Autodesk Inventor part; units mm, degrees
ref_plane "YZ Plane" through (0, 0, 0) normal (1, 0, 0) x (0, 1, 0)
ref_plane "XZ Plane" through (0, 0, 0) normal (0, 1, 0) x (-1, 0, 0)
ref_plane "XY Plane" through (0, 0, 0) normal (0, 0, 1) x (1, 0, 0)
sketch "Sketch1" plane through (0, 0, 0) normal (0, 0, 1) x (1, 0, 0)
  circle A0 centre (0, 0) radius 36
  dimension "d0" = 72
extrude "Extrusion1" add sketch "Sketch1" along normal blind 2
sketch "Sketch2" plane through (0, 0, 2) normal (0, 0, 1) x (1, 0, 0)
  circle A0 centre (0, 0) radius 36
  circle A1 centre (0, 0) radius 34
  dimension "d3" = 2
extrude "Extrusion2" add sketch "Sketch2" along normal blind 4
sketch "Sketch4" plane through (0, 0, 2) normal (0, 0, 1) x (1, 0, 0)
  point P0 (0, 0)
  point P1 (0, 0)
hole "Hole1" at (0, 0, 2) direction (0, 0, -1) diameter 10.1 end through all
sketch "Sketch5" plane through (0, 0, 2) normal (0, 0, 1) x (1, 0, 0)
  point P0 (0, 0)
  point P1 (0, 22.5)
  dimension "d13" = 22.5
hole "Hole2" at (0, 22.5, 2) direction (0, 0, -1) diameter 5.3 end through all
pattern_circular "Circular Pattern1" count 5 over 360 about axis through (0, 0, -100) along (0, 0, 1) of "Hole2"
sketch "Sketch8" plane through (0, 0, 2) normal (0, 0, 1) x (1, 0, 0)
  circle A0 centre (21.3988, 6.9529) radius 2.65
  circle A1 centre (13.2252, -18.2029) radius 2.65
  circle A2 centre (-13.2252, -18.2029) radius 2.65
  circle A3 centre (-21.3988, 6.9529) radius 2.65
  circle A4 centre (0, 22.5) radius 2.65
  circle A5 centre (0, 0) radius 5.05
  circle A6 centre (0, 0) radius 34
  line L0 (-2, 15) -> (2, 15)
  line L1 (2, 15) -> (2, 7)
  line L2 (2, 7) -> (-2, 7)
  line L3 (-2, 7) -> (-2, 15)
  dimension "d43" = 4
  dimension "d44" = 8
  dimension "d45" = 7
  dimension "d48" = 2
extrude "Extrusion5" cut sketch "Sketch8" against normal up to surface (2 mm away) draft 2 contours L0 L1 L2 L3
fillet "Fillet2" radius 0.25 4 edges at (0, 6.9302, 0) (2.0698, 11, 0) (0, 15.0698, 0) (-2.0698, 11, 0)
pattern_circular "Circular Pattern3" count 4 over 360 about axis through (0, 0, -100) along (0, 0, 1) of "Extrusion5", "Fillet2"
equation "\"d0\" = W_innerDiameter + W_wallThickness"
equation "\"d1\" = W_wallThickness"
equation "\"d3\" = W_wallThickness"
equation "\"d4\" = W_innerDepth"
equation "\"d6\" = W_innerGearHoleDiameter"
equation "\"d14\" = W_outerGearHoleDiameter"
equation "\"W_wallThickness\" = 2"
equation "\"W_innerDepth\" = 4"
equation "\"W_innerGearHoleDiameter\" = 10.1"
equation "\"W_outerGearHoleDiameter\" = 5.3"
equation "\"OG_distanceFromCenter\" = 22.5"
equation "\"W_innerDiameter\" = 70"
equation "\"Wheel_Related_W_\" = 0"
equation "\"W_holesClearance\" = 0.3"
equation "\"TempSpotReserved7\" = 0"
equation "\"TempSpotReserved8\" = 0"
equation "\"TempSpotReserved9\" = 0"
equation "\"TempSpotReserved10\" = 0"
equation "\"TempSpotReserved11\" = 0"
equation "\"TempSpotReserved12\" = 0"
equation "\"TempSpotReserved13\" = 0"
equation "\"TempSpotReserved14\" = 0"
equation "\"TempSpotReserved15\" = 0"
equation "\"TempSpotReserved16\" = 0"
equation "\"TempSpotReserved17\" = 0"
equation "\"TempSpotReserved18\" = 0"
equation "\"TempSpotReserved19\" = 0"
equation "\"TempSpotReserved20\" = 0"
equation "\"Inner_Gear_Related_IG_\" = 0"
equation "\"IG_shaftDiameter\" = 7.5"
equation "\"IG_shaftLength\" = 17"
equation "\"IG_gearThickness\" = 2"
equation "\"TempSpotReserved25\" = 0"
equation "\"TempSpotReserved26\" = 0"
equation "\"TempSpotReserved27\" = 0"
equation "\"TempSpotReserved28\" = 0"
equation "\"TempSpotReserved29\" = 0"
equation "\"TempSpotReserved30\" = 0"
equation "\"TempSpotReserved31\" = 0"
equation "\"TempSpotReserved32\" = 0"
equation "\"TempSpotReserved33\" = 0"
equation "\"TempSpotReserved34\" = 0"
equation "\"TempSpotReserved35\" = 0"
equation "\"TempSpotReserved36\" = 0"
equation "\"TempSpotReserved37\" = 0"
equation "\"TempSpotReserved38\" = 0"
equation "\"TempSpotReserved39\" = 0"
equation "\"TempSpotReserved40\" = 0"
equation "\"Outer_Gear_Related_OG_\" = 0"
equation "\"OG_shaftDiameter\" = 5"
equation "\"OG_gearDiameter\" = 25"
equation "\"OG_shaftLength\" = 9"
equation "\"OG_gearThickness\" = 2"
equation "\"TempSpotReserved47\" = 0"
equation "\"TempSpotReserved48\" = 0"
equation "\"TempSpotReserved49\" = 0"
equation "\"TempSpotReserved50\" = 0"
equation "\"TempSpotReserved51\" = 0"
equation "\"TempSpotReserved52\" = 0"
equation "\"TempSpotReserved53\" = 0"
equation "\"TempSpotReserved54\" = 0"
equation "\"TempSpotReserved55\" = 0"
equation "\"TempSpotReserved56\" = 0"
equation "\"TempSpotReserved57\" = 0"
equation "\"TempSpotReserved58\" = 0"
equation "\"TempSpotReserved59\" = 0"
equation "\"TempSpotReserved60\" = 0"
equation "\"Leg_Extensions_Related_LE_\" = 0"
equation "\"LE_baseDiameter\" = 5"
equation "\"LE_maxLength\" = 23.67256"
equation "\"LE_thickness\" = 2.5"
equation "\"IG_ratioToOuterGear\" = 1.25"
equation "\"B_bearingThickness\" = 1"
equation "\"TempSpotReserved43\" = 0"
equation "\"TempSpotReserved45\" = 0"
equation "\"Thisisatest\" = 25.4"
equation "\"TempSpotReserved46\" = 0"
equation "\"TempSpotReserved44\" = 0"
equation "\"LE_offsetAboveOuterGear\" = 0"
equation "\"Bearing_Related_B_\" = 0"
equation "\"TempSpotReserved42\" = 0"
equation "\"OG_skirtOffset\" = 5"
equation "\"OG_skirtThickness\" = 1"
equation "\"IG_skirtThickness\" = 2"
equation "\"IG_extentionLength\" = 19.5"
equation "\"IG_extentionThickness\" = 3"
equation "\"IG_slitWidth\" = 4"
equation "\"IG_slitlength\" = 8"
equation "\"IG_slitClearance\" = 0.2"
equation "\"IG_slitDistanceFromCenterHole\" = 7"
equation "\"Reserved_10\" = 0"
equation "\"Reserved_9\" = 0"
equation "\"Reserved_11\" = 0"
equation "\"Reserved_12\" = 0"
equation "\"Reserved_8\" = 0"
equation "\"Reserved_7\" = 0"
equation "\"Reserved_26\" = 0"
equation "\"Reserved_20\" = 0"
equation "\"Reserved_22\" = 0"
equation "\"Reserved_23\" = 0"
equation "\"Reserved_25\" = 0"
equation "\"Reserved_24\" = 0"
equation "\"Reserved_21\" = 0"
equation "\"Reserved_19\" = 0"
equation "\"Reserved_27\" = 0"
equation "\"Reserved_14\" = 0"
equation "\"Reserved_15\" = 0"
equation "\"Reserved_16\" = 0"
equation "\"Reserved_13\" = 0"
equation "\"Reserved_17\" = 0"
equation "\"Reserved_18\" = 0"
equation "\"Bearing_Related_BR_\" = 0"
equation "\"BR_bearingThickness\" = 1"
equation "\"Block_Related_BL_\" = 0"
equation "\"BL_width\" = 3.8"
equation "\"BL_length\" = 7.8"
equation "\"W_filletRadius\" = 0.25"
equation "\"W_extrutsionTaperAngle\" = 2deg"
equation "\"OG_protrudeDistance\" = 3"
equation "\"IG_dAxleDepth\" = 5"
equation "\"IG_dAxleShort\" = 1.5"
equation "\"IG_dAxleCircleDiameter\" = 2"
equation "\"IG_gearRatio\" = 1.25"
properties part number "wheel"
Geometry check sheet. Reference: the model listing, model coordinates, mm. A direction names the side the tool comes from. Round coordinates to 2 decimals unless told otherwise and drop trailing zeros. Order: outer loops, then holes, each group sorted by start corner. A loop starts at its lowest first (then second) coordinate and runs counter-clockwise, first axis right, second up. Notation, with made-up numbers: (89, 29.25) -> (117, 29.25) arc R31 ccw to (117, 63.25) -> close; hole circle Ø8 at (-28, -19). An arc over 180 degrees is marked (long way). Return JSON: item names as keys, results as strings. Group by question number.
Q1. Section check B-B, the plane y = 0. Record the boundary of the cut face in (x, z), plus the area to 3 significant figures.
Q2. Material ranges on probe 1 along X at (y, z) = (-1, 5.6); probe 2 along Y at (x, z) = (0, 0.9); probe 3 along Y at (x, z) = (19.5, 1.7), recorded low to high. Write a range as from..to.
Q3. Section check D-D, the plane z = 3.2. Record the boundary of the cut face in (x, y), plus the area to 3 significant figures.
Q4. Section check C-C, the plane y = -17. Record the boundary of the cut face in (x, z), plus the area to 3 significant figures.
Q5. Tool access check on faces 1 (the cylindrical face through (20.96, 4.34, 0.99)), 2 (the flat face through (7, -7, 2)). Record the directions out of +Z, -Z, +X, -X, +Y, -Y that give a thin tool (end or side, any length) a straight path to the whole face; none if there is none.
Q6. Section check A-A, the plane x = 0. Record the boundary of the cut face in (y, z).
Q7. Gauge pin test, flat ends, axial feed: pin 1 (13 mm diameter, centred on x = 0, y = 0, fed in from -Z); pin 2 (1.5 mm diameter, centred on x = 7, y = 8.5, fed in from +Z); pin 3 (1 mm diameter, centred on y = -20.5, z = 5.5, fed in from +X); pin 4 (2 mm diameter, centred on x = -15, z = 5, fed in from +Y). Record the tip position at first contact, or that the pin passes through.
Numbers:
{
 "1": {"outline": "(-36, 0) -> (-15.31, 0) arc R0.25 ccw to (-15.06, 0.24) -> (-15, 2) -> (-34, 2) -> (-34, 6) -> (-36, 6) -> close; (-7, 2) -> (-6.94, 0.24) arc R0.25 ccw to (-6.69, 0) -> (-5.05, 0) -> (-5.05, 2) -> close; (5.05, 0) -> (6.69, 0) arc R0.25 ccw to (6.94, 0.24) -> (7, 2) -> (5.05, 2) -> close; (15, 2) -> (15.06, 0.24) arc R0.25 ccw to (15.31, 0) -> (36, 0) -> (36, 6) -> (34, 6) -> (34, 2) -> close", "area": "107 mm^2"},
 "2": {"probe 1": "-35.99..-33.99, 33.99..35.99", "probe 2": "-36..-15.04, -6.96..-5.05, 5.05..6.96, 15.04..19.85, 25.15..36", "probe 3": "-30.26..5.1, 8.8..30.26"},
 "3": {"outline": "circle Ø72 at (0, 0); hole circle Ø68 at (0, 0)", "area": "440 mm^2"},
 "4": {"outline": "(-31.73, 0) -> (-15.59, 0) -> (-15.59, 2) -> (-29.44, 2) -> (-29.44, 6) -> (-31.73, 6) -> close; (-10.86, 0) -> (10.86, 0) -> (10.86, 2) -> (-10.86, 2) -> close; (15.59, 0) -> (31.73, 0) -> (31.73, 6) -> (29.44, 6) -> (29.44, 2) -> (15.59, 2) -> close", "area": "126 mm^2"},
 "5": {"face 1": "+Z, -Z", "face 2": "+Z"},
 "6": {"outline": "(-36, 0) -> (-15.31, 0) arc R0.25 ccw to (-15.06, 0.24) -> (-15, 2) -> (-34, 2) -> (-34, 6) -> (-36, 6) -> close; (-7, 2) -> (-6.94, 0.24) arc R0.25 ccw to (-6.69, 0) -> (-5.05, 0) -> (-5.05, 2) -> close; (5.05, 0) -> (6.69, 0) arc R0.25 ccw to (6.94, 0.24) -> (7, 2) -> (5.05, 2) -> close; (15, 2) -> (15.06, 0.24) arc R0.25 ccw to (15.31, 0) -> (19.85, 0) -> (19.85, 2) -> close; (25.15, 0) -> (36, 0) -> (36, 6) -> (34, 6) -> (34, 2) -> (25.15, 2) -> close"},
 "7": {"pin 1": "z = 0", "pin 2": "z = 2", "pin 3": "x = 29.93", "pin 4": "y = 33.17"}
}
